Could you check a few things on this drawing? It's one solid part, dimensions in mm from its lowest x, y, z. A direction names the side the tool comes from. Give positions to 0.01 mm unless a question says otherwise; leave off trailing zeros. Loops run counter-clockwise (first coordinate to the right, second up) from the corner with the lowest first, then second, coordinate; pieces in that order, holes last. Notation, with made-up numbers: (49.25, 22) -> (67.25, 22) arc R27 cw to (67.25, 38) -> close; hole circle Ø4 at (-4, -0.75). An arc over 180 degrees is marked (long way). Use CSV: the item, a comma, the result in double quotes.
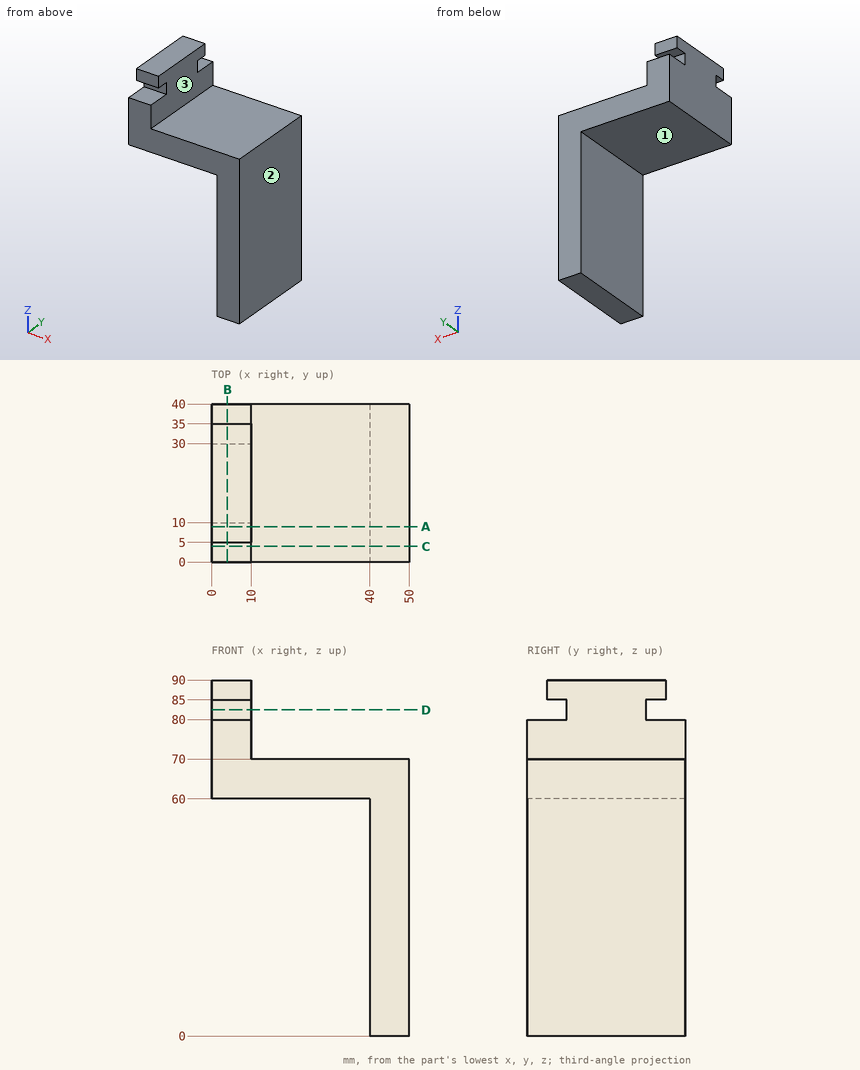
(1) If we section it at C-C, the plane y = 4: Write out the boundary of the cut face in (x, z), then the cut area to 3 significant figures.
Answer sheet:
outline,"(0, 60) -> (40, 60) -> (40, 0) -> (50, 0) -> (50, 70) -> (10, 70) -> (10, 80) -> (0, 80) -> close"
area,"1,200 mm2"
(2) If we section it at B-B, the plane x = 4: Write out the boundary of the cut face in (y, z), then the cut area to 3 significant figures.
Answer sheet:
outline,"(0, 60) -> (40, 60) -> (40, 80) -> (30, 80) -> (30, 85) -> (35, 85) -> (35, 90) -> (5, 90) -> (5, 85) -> (10, 85) -> (10, 80) -> (0, 80) -> close"
area,"1,050 mm2"
(3) Which directions (+Z, -Z, +X, -X, +Y, -Y) give clear straight access to the entire face, cutting with the end or side of a thin tool? Please do the marked faces 1, 2 and 3.
Answer sheet:
face 1,"-Z, -X, +Y, -Y"
face 2,"+Z, -Z, +X, +Y, -Y"
face 3,"+Z, +X, +Y, -Y"
(4) If we section it at D-D, the plane z = 82.5: Write out the boundary of the cut face in (x, y).
Answer sheet:
outline,"(0, 10) -> (10, 10) -> (10, 30) -> (0, 30) -> close"
(5) If I drill on L1, parallel to Z at x = 46, y = 4.5; L2, parallel to Z at x = 23.5, y = 8; L3, parallel to X at y = 14, z = 54, over which ranges is the centre line in solid material (lowest first)? Write a range as from..to.
Answer sheet:
L1,"z = 0..70"
L2,"z = 60..70"
L3,"x = 40..50"
(6) If we section it at A-A, the plane y = 9: Write out the boundary of the cut face in (x, z).
Answer sheet:
outline,"(0, 60) -> (40, 60) -> (40, 0) -> (50, 0) -> (50, 70) -> (10, 70) -> (10, 80) -> (0, 80) -> close; (0, 85) -> (10, 85) -> (10, 90) -> (0, 90) -> close"
(7) Will these pins go through, and if not, where does the flat tip stop? pin 1 Ø4 at (x, y) = (7, 8.5) entering from -Z; pin 2 Ø1.5 at (x, z) = (7, 87.5) entering from +Y; pin 3 Ø5.5 at (x, z) = (3, 88) entering from -Y.
Answer sheet:
pin 1,"stops at z = 60"
pin 2,"stops at y = 35"
pin 3,"stops at y = 5"
